from build123d import *

# Parameters (mm, degrees)
F0_R     = 11.2014
F1_DEPTH = 10.47496
F2_R     = 7.9375
F3_DEPTH = 9.525
F5_D     = 10.1
F6_SIZE  = 1


with BuildPart() as f1:
    # F0 (on Right) → F1 (new body)
    with BuildSketch(Plane.YZ):
        Circle(F0_R)
    extrude(amount=F1_DEPTH)

    # F2 (on face) → F3 (join)
    with BuildSketch(Plane.YZ.offset(10.47496)):
        Circle(F2_R)
    extrude(amount=F3_DEPTH)

    # F5 (through all)
    with Locations(Plane.YZ.offset(19.99996)):
        with Locations((0, 0)):
            Hole(F5_D / 2)

    # F6
    f6_edges = [f1.edges().sort_by_distance(p)[0] for p in [
        (19.99996, -7.9375, 0),
    ]]
    chamfer(f6_edges, length=F6_SIZE)


solid = f1.part
The model under review builds one solid part; all positions refer to its coordinate system, in mm. A direction names the side the tool comes from. Coordinates: 2 decimals unless noted, no trailing zeros. Loops run counter-clockwise (first coordinate to the right, second up) from the corner with the lowest first, then second, coordinate; pieces in that order, holes last. Notation, with made-up numbers: M 16,1.25 L 67,1.25 A19 ccw 67,31.25 Z; hole C 13.25,62 d11. An arc over 180 degrees is marked long. Put each result on its own line as item: value. Start each with the question number.
Q1. Wall thickness on line 1 (Z direction, x = 10.75, y = 0); line 2 (X direction, y = -5.5, z = 6.5); line 3 (Y direction, x = 4, z = -1): over which ranges is each line inside the solid? List them lowest first.
Q2. Clearance check with flat-ended pins moving along their axes: pin 1 (2 mm diameter, centred on x = 13, y = -6, fed in from +Z); pin 2 (5 mm diameter, centred on x = 14.5, z = -1, fed in from -Y). State where each tip first meets the part, or that it passes through.
Q3. Add section A-A (y = 0). Write out the cut boundary in (x, z).
Q4. For faces 1 (the cylindrical face through (14.68, -1.72, -7.75)), 2 (the flat face through (0, 5, -2)), list the 3-axis set-ups (+Z, -Z, +X, -X, +Y, -Y) from which the entire face can be reached by the end or side of a thin tool; tool diameter is ignored.
Q5. Add section D-D (x = 1.5). Write out the cut boundary in (y, z), and give its area (3 significant figures).
Q6. The part is to be moulded in two halves that separate along Y. For faces 3 (the flat face through (10.475, 2, 8)), 4 (the cylindrical face through (9.86, -4.817, 1.517)), 5 (the cylindrical face through (5.16, -11.19, 0.49)), say which applies: +Y half, -Y half, draft (parallel to the pull), parting line (faces both ways), or undercut.
Answers:
1. line 1: z = -7.94 to -5.05, 5.05 to 7.94
1. line 2: x = 0 to 10.47
1. line 3: y = -11.16 to -4.95, 4.95 to 11.16
2. pin 1: stops at z = 6.16
2. pin 2: stops at y = -7.94
3. outline: M 0,-11.2 L 10.47,-11.2 L 10.47,-7.94 L 19,-7.94 L 20,-6.94 L 20,-5.05 L 0,-5.05 Z; M 0,5.05 L 20,5.05 L 20,6.94 L 19,7.94 L 10.47,7.94 L 10.47,11.2 L 0,11.2 Z
4. face 1: +X
4. face 2: +Z, -Z, -X, +Y, -Y
5. outline: C 0,0 d22.4; hole C 0,0 d10.1
5. area: 314 mm^2
6. face 3: draft
6. face 4: undercut
6. face 5: parting line
